from build123d import *

# Parameters (mm, degrees)
F0_W     = 711.2
F0_H     = 84.1375
F2_W     = 44.45
F2_H     = 44.45
F3_DEPTH = 25.4
F4_W     = 44.45
F4_H     = 44.45
F5_DEPTH = 25.4


with BuildPart() as f1:
    # F0 (on Top) → F1 (revolve)
    with BuildSketch(Plane.XY):
        with Locations((0, 42.06875)):
            Rectangle(F0_W, F0_H)
        with BuildLine():
            add(Edge.make_bspline(
                [(495.3, 44.45), (491.1825215885, 44.0904084612), (479.4418370711, 43.0650598398), (427.3573599541, 55.187373247), (400.0577825465, 83.2970238087), (370.6219245107, 83.8535099048), (355.6, 84.1375)],
                knots=[0, 0, 0, 0, 0.1628231526, 0.4642781518, 0.7266064691, 1, 1, 1, 1], degree=3))
            Line((355.6, 84.1375), (355.6, 0))
            Line((355.6, 0), (495.3, 0))
            Line((495.3, 0), (495.3, 44.45))
        make_face()
        with BuildLine():
            Line((-355.6, 0), (-355.6, 84.1375))
            add(Edge.make_bspline(
                [(-495.3, 44.45), (-491.1825215885, 44.0904084612), (-479.4418370711, 43.0650598398), (-427.3573599541, 55.187373247), (-400.0577825465, 83.2970238087), (-370.6219245107, 83.8535099048), (-355.6, 84.1375)],
                knots=[0, 0, 0, 0, 0.1628231526, 0.4642781518, 0.7266064691, 1, 1, 1, 1], degree=3))
            Line((-495.3, 44.45), (-495.3, 0))
            Line((-495.3, 0), (-355.6, 0))
        make_face()
    revolve(axis=Axis((0, 0, 0), (1, 0, 0)))

    # F2 (on face) → F3 (cut)
    with BuildSketch(Plane(origin=(-495.3, 0, 0), x_dir=(0, -1, 0), z_dir=(-1, 0, 0))):
        Rectangle(F2_W, F2_H)
    extrude(amount=-F3_DEPTH, mode=Mode.SUBTRACT)

    # F4 (on face) → F5 (cut)
    with BuildSketch(Plane.YZ.offset(495.3)):
        Rectangle(F4_W, F4_H)
    extrude(amount=-F5_DEPTH, mode=Mode.SUBTRACT)


solid = f1.part
Work out the finished part from the listing and answer in its coordinate system (mm). A direction names the side the tool comes from. Coordinates: 2 decimals unless noted, no trailing zeros. Loops run counter-clockwise (first coordinate to the right, second up) from the corner with the lowest first, then second, coordinate; pieces in that order, holes last. Notation, with made-up numbers: (65, 88.5) -> (121, 88.5) arc R15 cw to (121, 102.5) -> close; hole circle Ø3 at (83.5, 6). An arc over 180 degrees is marked (long way). Answer as CSV lines item,"result".
1) Flat-ended cylindrical pins translate along their axes: pin 1 (8 mm diameter, centred on x = -53, z = 12.5, fed in from -Y); pin 2 (20.5 mm diameter, centred on x = -485.5, y = 6, fed in from +Z); pin 3 (12.5 mm diameter, centred on x = 479.5, z = 6, fed in from +Y). Find the tip coordinate at first contact, or state that the pin passes through.
A:
pin 1,"stops at y = -83.71"
pin 2,"stops at z = 44.95"
pin 3,"stops at y = 45.21"
2) Straight lines are drawn through the part: probe 1 along Z at (x, y) = (376, 76); probe 2 along Y at (x, z) = (-80, 37.5); probe 3 along Y at (x, z) = (392.5, 17). For each, find the intervals that lie inside material, in ascending order.
A:
probe 1,"z = -34.12 to 34.12"
probe 2,"y = -75.32 to 75.32"
probe 3,"y = -78.67 to 78.67"
3) The part is cut by section A-A (x = 165.5). Give the vertices of the cut face in (y, z) (1 decimal), and give its area (3 significant figures).
A:
outline,"circle Ø168.3 at (0, 0)"
area,"22,200 mm²"
4) For a pull along Y with two mould halves and no side action, classify faces 1 (the face through (495.3, 1, -29)), 2 (the face through (4.978, -18.239, -82.137)), 3 (the face through (483, 0, -22.225)) as released by +Y, released by -Y, zero draft, split by the parting line, or undercut.
A:
face 1,"zero draft"
face 2,"split by the parting line"
face 3,"undercut"
5) For faces 4 (the face through (-483, 0, 22.225)), 5 (the face through (469.9, 0, 0)), 6 (the face through (-495.3, -1, -29)), determine the directions among +Z, -Z, +X, -X, +Y, -Y from which every point of the face is accessible in a straight line to the end or side of a thin tool.
A:
face 4,"-X"
face 5,"+X"
face 6,"+Z, -Z, -X, +Y, -Y"
